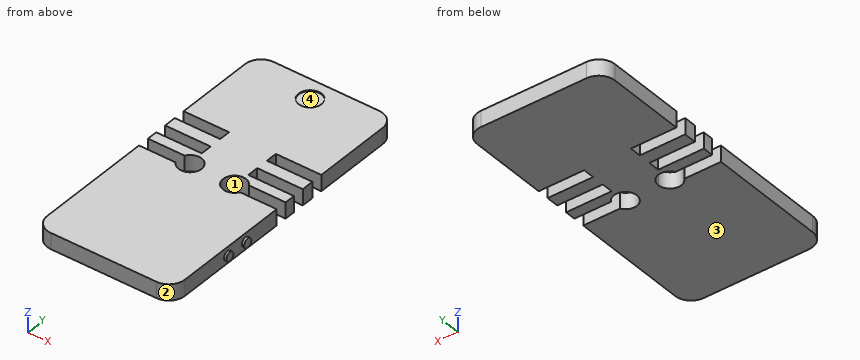
from build123d import *

# Parameters (mm, degrees)
F0_W      = 60
F0_H      = 125
F1_DEPTH  = 7
F2_R      = 7
F3_R      = 7
F4_R      = 7
F5_R      = 2
F6_DEPTH  = 1
F9_W      = 20
F9_H      = 5
F10_DEPTH = 88.1
F7_R      = 5
F12_DEPTH = 0.4


# Not quite as in the source:
# - the program builds the solid bodies; features that only make, move or delete a surface that nothing else refers to are left out


with BuildPart() as f1:
    # F0 (on Top) → F1 (new body)
    with BuildSketch(Plane.XY):
        with Locations((4.798640497, -0.129804003)):
            Rectangle(F0_W, F0_H)
    extrude(amount=F1_DEPTH)

    # F2
    f2_edges = [f1.edges().sort_by_distance(p)[0] for p in [
        (-25.20136, -62.629804, 3.5),
    ]]
    fillet(f2_edges, radius=F2_R)

    # F3
    f3_edges = [f1.edges().sort_by_distance(p)[0] for p in [
        (-25.20136, 62.370196, 3.5),
        (34.79864, -62.629804, 3.5),
    ]]
    fillet(f3_edges, radius=F3_R)

    # F4
    f4_edges = [f1.edges().sort_by_distance(p)[0] for p in [
        (34.79864, 62.370196, 3.5),
    ]]
    fillet(f4_edges, radius=F4_R)

    # F5 (on face) → F6 (join)
    with BuildSketch(Plane.YZ.offset(34.798640497)):
        with Locations((-31.6818073764, 3.2178394031)):
            Circle(F5_R)
        with Locations((-21.6818073764, 3.2178394031)):
            Circle(F5_R)
    extrude(amount=F6_DEPTH)

    # F9 (on Top) → F10 (cut)
    with BuildSketch(Plane.XY):
        with Locations((-15.4034045642, 18.4103432111)):
            Rectangle(F9_W, F9_H)
        with Locations((24.9580888633, 18.4103432111)):
            Rectangle(F9_W, F9_H)
        with Locations((-15.3402814512, 8.0003063194)):
            Rectangle(F9_W, F9_H)
        with Locations((24.940414155, 8.0003063194)):
            Rectangle(F9_W, F9_H)
        with BuildLine():
            Line((-9.2095649145, 0.8613835648), (-25.9844651689, 0.8613835648))
            Line((-25.9844651689, 0.8613835648), (-25.9844651689, -4.1386164352))
            Line((-25.9844651689, -4.1386164352), (-9.2095649145, -4.1386164352))
            ThreePointArc((-9.2095649145, -4.1386164352), (-9.8794378956, -1.6386164352), (-9.2095649145, 0.8613835648))
        make_face()
        with BuildLine():
            ThreePointArc((0.1205621044, -1.6386164352), (-3.5853426701, 3.1910126962), (-9.2095649145, 0.8613835648))
            ThreePointArc((-9.2095649145, 0.8613835648), (-9.8794378956, -1.6386164352), (-9.2095649145, -4.1386164352))
            ThreePointArc((-9.2095649145, -4.1386164352), (-3.5853426701, -6.4682455667), (0.1205621044, -1.6386164352))
        make_face()
        with BuildLine():
            Line((36.6257494559, -4.1386164352), (36.6257494559, 0.8613835648))
            Line((36.6257494559, 0.8613835648), (18.8484872035, 0.8613835648))
            ThreePointArc((18.8484872035, 0.8613835648), (9.5183601846, -1.6386164352), (18.8484872035, -4.1386164352))
            Line((18.8484872035, -4.1386164352), (36.6257494559, -4.1386164352))
        make_face()
    extrude(amount=F10_DEPTH, mode=Mode.SUBTRACT)

    # F7 (on face) → F12 (cut)
    with BuildSketch(Plane.XY.offset(7)):
        with Locations((4.798640497, 53.2364137471)):
            Circle(F7_R)
    extrude(amount=-F12_DEPTH, mode=Mode.SUBTRACT)


solid = f1.part
The model under review builds one solid part; all positions refer to its coordinate system, in mm. Face numbers are marked on the shaded views. Coordinates: 2 decimals unless noted, no trailing zeros. Order: outer loops, then holes, each group sorted by start corner. A loop starts at its lowest first (then second) coordinate and runs counter-clockwise, first axis right, second up. Notation, with made-up numbers: (64, 80) -> (104, 80) arc R15 cw to (104, 87) -> close; hole circle Ø5 at (20, 16). An arc over 180 degrees is marked (long way). Answer in a Markdown table with one row per item.
(1) Insertion check: pin 1 (1.5 mm diameter, centred on y = 19, z = 4.5, fed in from -X); pin 2 (2.5 mm diameter, centred on y = 18, z = 3.5, fed in from +X). Each pin has a flat end and moves straight along its axis. Give the tip position at first contact, or say it passes through.
Answers:
| item | result |
|---|---|
| pin 1 | x = -5.4 |
| pin 2 | x = 14.96 |
(2) Consider section B-B (y = -52). Write out the cut boundary in (x, z).
Answers:
| item | result |
|---|---|
| outline | (-25.2, 0) -> (34.8, 0) -> (34.8, 7) -> (-25.2, 7) -> close |
(3) Wall thickness on line 1 along Y through (x, z) = (-12.5, 6.5); line 2 along Y through (x, z) = (29, 5); line 3 along Y through (x, z) = (14.5, 5.5): over which ranges is each line inside the solid? List them lowest first.
Answers:
| item | result |
|---|---|
| line 1 | -62.63 to -4.14, 0.86 to 5.5, 10.5 to 15.91, 20.91 to 62.37 |
| line 2 | -62.53 to -4.14, 0.86 to 5.5, 10.5 to 15.91, 20.91 to 62.27 |
| line 3 | -62.63 to -6.64, 3.36 to 62.37 |
(4) Consider section A-A (x = -12). Write out the cut boundary in (y, z), plus the area to 3 significant figures.
Answers:
| item | result |
|---|---|
| outline | (-62.63, 0) -> (-4.14, 0) -> (-4.14, 7) -> (-62.63, 7) -> close; (0.86, 0) -> (5.5, 0) -> (5.5, 7) -> (0.86, 7) -> close; (10.5, 0) -> (15.91, 0) -> (15.91, 7) -> (10.5, 7) -> close; (20.91, 0) -> (62.37, 0) -> (62.37, 7) -> (20.91, 7) -> close |
| area | 770 mm² |
(5) The part is to be moulded in two halves that separate along X. For the marked faces 1, 2, 3 and 4, say which applies: +X half, -X half, draft (parallel to the pull), parting line (faces both ways), or undercut.
Answers:
| item | result |
|---|---|
| face 1 | undercut |
| face 2 | +X half |
| face 3 | draft |
| face 4 | undercut |
(6) Consider section C-C (x = -20). Write out the cut boundary in (y, z).
Answers:
| item | result |
|---|---|
| outline | (-62.39, 0) -> (-4.14, 0) -> (-4.14, 7) -> (-62.39, 7) -> close; (0.86, 0) -> (5.5, 0) -> (5.5, 7) -> (0.86, 7) -> close; (10.5, 0) -> (15.91, 0) -> (15.91, 7) -> (10.5, 7) -> close; (20.91, 0) -> (62.14, 0) -> (62.14, 7) -> (20.91, 7) -> close |
